Part model, mm, in its own coordinate system. A direction names the side the tool comes from. Give positions to 0.01 mm unless a question says otherwise; leave off trailing zeros. Order: outer loops, then holes, each group sorted by start corner. A loop starts at its lowest first (then second) coordinate and runs counter-clockwise, first axis right, second up. Notation, with made-up numbers: M -21,8 L 38,8 A31 ccw 38,39 Z; hole C 67.25,82.5 d6. An arc over 180 degrees is marked long. Answer as a JSON object with one key per item and string values.
Autodesk Inventor part; units mm, degrees
ref_plane "Work Plane2" through (40.95, 3.5, 3.25) normal (-0.9659258, -0.258819, 0) x (0, 0, 1)
ref_plane "YZ Plane" through (0, 0, 0) normal (1, 0, 0) x (0, 1, 0)
ref_plane "XZ Plane" through (0, 0, 0) normal (0, 1, 0) x (-1, 0, 0)
sketch "Sketch1" plane through (0, 0, 0) normal (0, 0, 1) x (1, 0, 0)
  line L0 (0, 0) -> (88.9, 0)
  line L1 (88.9, 0) -> (88.9, 3.5)
  line L2 (88.9, 3.5) -> (0, 3.5)
  line L3 (0, 3.5) -> (0, 0)
  line L4 (0, 92.4) -> (50.8, 92.4)
  line L5 (50.8, 92.4) -> (50.8, 97.4)
  line L6 (50.8, 97.4) -> (0, 97.4)
  line L7 (0, 97.4) -> (0, 92.4)
  arc A0 (0, 92.4) -> (0, 3.5) centre (0, 47.95) ccw
  arc A1 (0, 97.4) -> (0, 0) centre (0, 48.7) ccw
  dimension "d0" = 88.9
  dimension "d1" = 3.5
  dimension "d2" = 50.8
  dimension "d3" = 5
  dimension "d4" = 88.9
extrude "Extrusion1" add sketch "Sketch1" along normal blind 20
sketch "Sketch2" plane through (0, 3.5, 0) normal (0, 1, 0) x (1, 0, 0)
  line L0 (88.9, 0) -> (0, 0)
  line L1 (0, 0) -> (0, -20)
  line L2 (88.9, -20) -> (0, -20)
  line L3 (88.9, 0) -> (88.9, -20)
sketch "Sketch3" plane through (0, 92.4, 0) normal (0, -1, 0) x (1, 0, 0)
  line L0 (0, 0) -> (0, 20)
  line L1 (47.95, 6.5) -> (40.95, 6.5)
  line L2 (40.95, 6.5) -> (40.95, 13.5)
  line L3 (40.95, 13.5) -> (47.95, 13.5)
  line L4 (47.95, 13.5) -> (47.95, 6.5)
  line L5 (47.95, 6.5) -> (40.95, 13.5) construction
  line L6 (40.95, 6.5) -> (47.95, 13.5) construction
  point P0 (44.45, 10)
  dimension "d8" = 7
  dimension "d9" = 7
  dimension "d10" = 44.45
extrude "Extrusion2" cut sketch "Sketch3" against normal blind 3
ref_plane "Work Plane1" through (40.95, 95.4, 6.5) normal (-0.8660254, 0.5, 0) x (0, 0, 1)
sketch "Sketch4" plane through (40.95, 95.4, 6.5) normal (-0.8660254, 0.5, 0) x (0, 0, 1)
  line L0 (0, 0) -> (7, 0)
  line L1 (-6.5, -104.4399) -> (13.5, -104.4399)
  line L2 (13.5, -104.4399) -> (13.5, -108.0877)
  line L3 (13.5, -108.0877) -> (-6.5, -108.0877)
  line L4 (-6.5, -108.0877) -> (-6.5, -104.4399)
  line L5 (13.5, -3.4641) -> (-6.5, -3.4641)
  line L6 (-6.5, -3.4641) -> (-6.5, 2.3094)
  line L7 (-6.5, 2.3094) -> (13.5, 2.3094)
  line L8 (13.5, 2.3094) -> (13.5, -3.4641)
  line L9 (7, 0) -> (0, 0)
  line L10 (0, 0) -> (0, -3)
  line L11 (0, -3) -> (7, -3)
  line L12 (7, -3) -> (7, 0)
  point P0 (-6.5, -103.0938)
  dimension "d14" = 3
extrude "Extrusion3" cut sketch "Sketch4" along normal through all both and the other way through all contours L0 L12 L11 L10
sketch "Sketch5" plane through (0, 3.5, 0) normal (0, 1, 0) x (1, 0, 0)
  line L0 (0, 0) -> (0, -20)
  line L1 (47.95, -13.5) -> (40.95, -13.5)
  line L2 (40.95, -13.5) -> (40.95, -6.5)
  line L3 (40.95, -6.5) -> (47.95, -6.5)
  line L4 (47.95, -6.5) -> (47.95, -13.5)
  line L5 (47.95, -13.5) -> (40.95, -6.5) construction
  line L6 (40.95, -13.5) -> (47.95, -6.5) construction
  line L7 (38.45, -16) -> (50.45, -16)
  line L8 (50.45, -16) -> (50.45, -4)
  line L9 (50.45, -4) -> (38.45, -4)
  line L10 (38.45, -4) -> (38.45, -16)
  line L11 (38.45, -16) -> (50.45, -4) construction
  line L12 (50.45, -16) -> (38.45, -4) construction
  point P0 (44.45, -10)
  dimension "d17" = 7
  dimension "d18" = 7
  dimension "d19" = 44.45
  dimension "d20" = 12
  dimension "d21" = 12
extrude "Extrusion4" add sketch "Sketch5" along normal blind 3
ref_plane "Work Plane2" through (40.95, 3.5, 3.25) normal (-0.9659258, -0.258819, 0) x (0, 0, 1)
sketch "Sketch6" plane through (40.95, 3.5, 3.25) normal (-0.9659258, -0.258819, 0) x (0, 0, 1)
  line L0 (10.25, 0) -> (3.25, 0)
  line L1 (16.75, -3.6235) -> (-3.25, -3.6235)
  line L2 (-3.25, -3.6235) -> (-3.25, 0)
  line L3 (-3.25, 0) -> (0.75, 0)
  line L4 (0.75, 0) -> (0.75, 3.1058)
  line L5 (0.75, 3.1058) -> (12.75, 3.1058)
  line L6 (12.75, 3.1058) -> (12.75, 0)
  line L7 (12.75, 0) -> (16.75, 0)
  line L8 (16.75, 0) -> (16.75, -3.6235)
  line L9 (16.75, 92.0361) -> (-3.25, 92.0361)
  line L10 (-3.25, 92.0361) -> (-3.25, 97.2124)
  line L11 (-3.25, 97.2124) -> (16.75, 97.2124)
  line L12 (16.75, 97.2124) -> (16.75, 92.0361)
  line L13 (10.25, 0) -> (3.25, 0)
  line L14 (3.25, 0) -> (3.25, 3.1058)
  line L15 (3.25, 3.1058) -> (10.25, 3.1058)
  line L16 (10.25, 3.1058) -> (10.25, 0)
  point P0 (-3.25, 7.2179)
extrude "Extrusion5" cut sketch "Sketch6" along normal through all both and the other way through all contours L0 L14 L5 L16
sketch "Sketch7" plane through (0, 6.5, 0) normal (0, 1, 0) x (1, 0, 0)
  line L0 (40.1462, -13.5) -> (40.1462, -6.5)
  line L1 (38.45, -4) -> (38.45, -16)
  line L2 (38.45, -16) -> (38.45, -4)
  line L3 (38.45, -4) -> (50.45, -4)
  line L4 (50.45, -4) -> (50.45, -6.5)
  line L5 (50.45, -6.5) -> (40.1462, -6.5)
  line L6 (40.1462, -6.5) -> (40.1462, -13.5)
  line L7 (40.1462, -13.5) -> (50.45, -13.5)
  line L8 (50.45, -13.5) -> (50.45, -16)
  line L9 (50.45, -16) -> (38.45, -16)
  line L10 (-16.053, 0) -> (-16.053, -20)
  line L11 (-16.053, -20) -> (-24.3074, -20)
  line L12 (-24.3074, -20) -> (-24.3074, 0)
  line L13 (-24.3074, 0) -> (-16.053, 0)
  line L14 (40.1462, -13.5) -> (38.45, -13.5)
  line L15 (40.1462, -6.5) -> (38.45, -6.5)
  point P0 (0, 0)
extrude "Extrusion6" cut sketch "Sketch7" against normal blind 3 contours L14 L1 L15 L0
sketch "Sketch8" plane through (0, 0, 0) normal (0, -1, 0) x (1, 0, 0)
  line L0 (27.8878, 13.5) -> (27.8878, 6.5)
  line L1 (27.8878, 6.5) -> (15.8878, 6.5)
  line L2 (15.8878, 6.5) -> (15.8878, 13.5)
  line L3 (15.8878, 13.5) -> (27.8878, 13.5)
  line L4 (15.8878, 13.5) -> (-12.9863, 13.5)
  line L5 (-12.9863, 13.5) -> (-12.9863, 6.5)
  line L6 (-12.9863, 6.5) -> (15.8878, 6.5)
  line L7 (15.8878, 6.5) -> (15.8878, 13.5)
extrude "Extrusion7" cut sketch "Sketch8" against normal blind 1.5
properties part number "PinewoodFinish"
1. Cut at C-C on y = 31. Give the cut face in (x, z), plus the area to 3 significant figures.
Worked answers:
{"outline": "M -45.37,0 L -41.09,0 L -41.09,20 L -45.37,20 Z", "area": "85.6 mm^2"}
2. Probe line 1 along Y through (x, z) = (24, 2); line 2 along Y through (x, z) = (30.5, 10.5); line 3 along Y through (x, z) = (67, 6.75). List the from-to ranges inside material, lowest first.
Worked answers:
{"line 1": "y = 0 to 3.5, 92.4 to 97.4", "line 2": "y = 0 to 0.7, 92.4 to 97.4", "line 3": "y = 0 to 3.5"}
3. Cut at B-B on z = 17.5. Give the cut face in (x, y).
Worked answers:
{"outline": "M 0,0 L 88.9,0 L 88.9,3.5 L 0,3.5 A44.45 cw 0,92.4 L 50.8,92.4 L 50.8,97.4 L 0,97.4 A48.7 ccw Z"}
4. Two-plate mould, pull along Z, no slides. Class faces 1 (the flat face through (25, 2, 13.5)), 2 (the flat face through (88.9, 2, 10)), 3 (the flat face through (44, 95.4, 10)), 4 (the flat face through (-16, 6, 0)): +Z half, -Z half, draft (parallel to the pull), parting line (faces both ways), or undercut.
Worked answers:
{"face 1": "undercut", "face 2": "draft", "face 3": "undercut", "face 4": "-Z half"}
5. Pin check, flat tips, straight feed: P1, Ø0.9, axis at x = 42, y = 5.5, coming from the -Z side; P2, Ø2.5, axis at y = 95.5, z = 13.5, coming from the +X side; P3, Ø2, axis at x = 7, z = 9, coming from the -Y side; P4, Ø5, axis at x = 32, y = 3, coming from the -Z side. Stop position of each tip, or through.
Worked answers:
{"P1": "stops at z = 4", "P2": "stops at x = 50.8", "P3": "stops at y = 1.5", "P4": "stops at z = 0"}
6. Cut at A-A on x = -24. Give the cut face in (y, z), plus the area to 3 significant figures.
Worked answers:
{"outline": "M 6.32,0 L 10.54,0 L 10.54,20 L 6.32,20 Z; M 85.36,0 L 91.08,0 L 91.08,20 L 85.36,20 Z", "area": "198 mm^2"}
7. Cut at D-D on x = 56. Give the cut face in (y, z), plus the area to 3 significant figures.
Worked answers:
{"outline": "M 0,0 L 3.5,0 L 3.5,20 L 0,20 Z", "area": "70.0 mm^2"}
8. Which spindle directions (+Z, -Z, +X, -X, +Y, -Y) get a long thin tool onto all of the face, cutting with end or side? Do faces 5 (the flat face through (50.8, 95, 10)), 6 (the flat face through (50.45, 5, 10)), 7 (the flat face through (35.877, 94.865, 9.951)). Say none if no direction does.
Worked answers:
{"face 5": "+Z, -Z, +X, +Y", "face 6": "+Z, -Z, +X", "face 7": "none"}
